Can you work these out from the drawing? Everything is in mm from the part's minimum corner. A direction names the side the tool comes from. Coordinates: 2 decimals unless noted, no trailing zeros. Loops run counter-clockwise (first coordinate to the right, second up) from the corner with the lowest first, then second, coordinate; pieces in that order, holes last. Notation, with made-up numbers: (-31.75, 88) -> (17.25, 88) arc R27 cw to (17.25, 117) -> close; hole circle Ø4 at (-34, 65.5). An arc over 180 degrees is marked (long way). Put each result on its own line as item: value. Start each with the question number.
Item 1: Will these pins go through, and if not, where does the flat tip stop? P1, Ø1.5, axis at x = 14, z = 3, coming from the +Y side; P2, Ø2, axis at x = 8, z = 6, coming from the -Y side.
Item 2: We'd pull the mould along Z, two halves only. Please class the marked faces 1, 2, 3 and 4: pulls with the +Z half, pulls with the -Z half, needs draft (parallel to the pull), parting line crosses it, or undercut.
Item 3: For the marked faces 5 and 6, which set-ups out of +Z, -Z, +X, -X, +Y, -Y let a thin tool reach every point of the face, with its end or its side?
Item 4: If we section it at C-C on y = 11.25: Please give me the cut outline in (x, z) (1 decimal).
Item 5: If we section it at B-B on y = 16.5: Please give me the cut outline in (x, z) (1 decimal).
Item 6: If we section it at D-D on x = 14.75: Please give me the cut outline in (y, z) (1 decimal).
Item 7: Please list where these lines run through material, in increasing order: L1, parallel to Z at x = 2.75, y = 13.5 (1 decimal); L2, parallel to Y at x = 9, z = 0.5 (1 decimal); L3, parallel to X at y = 10.25, z = 4.5 (1 decimal). Write a range as from..to.
Item 8: If we section it at A-A on x = 10.25: Please give me the cut outline in (y, z) (1 decimal).
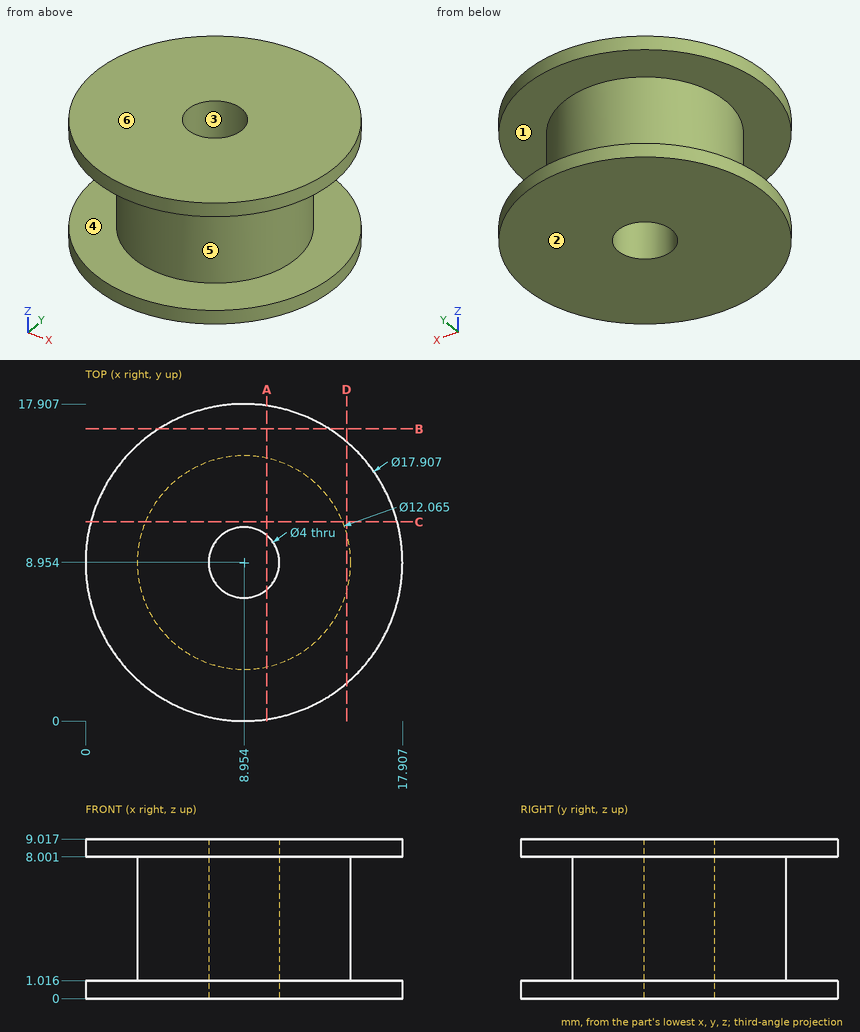
Solutions:
1. P1: y = 13.19
1. P2: y = 2.92
2. face 1: undercut
2. face 2: pulls with the -Z half
2. face 3: needs draft
2. face 4: undercut
3. face 5: none
3. face 6: +Z, +X, -X, +Y, -Y
4. outline: (0.3, 0) -> (17.6, 0) -> (17.6, 1) -> (14.5, 1) -> (14.5, 8) -> (17.6, 8) -> (17.6, 9) -> (0.3, 9) -> (0.3, 8) -> (3.4, 8) -> (3.4, 1) -> (0.3, 1) -> close
5. outline: (4.1, 0) -> (13.8, 0) -> (13.8, 1) -> (4.1, 1) -> close; (4.1, 8) -> (13.8, 8) -> (13.8, 9) -> (4.1, 9) -> close
6. outline: (2.1, 0) -> (15.8, 0) -> (15.8, 1) -> (10.6, 1) -> (10.6, 8) -> (15.8, 8) -> (15.8, 9) -> (2.1, 9) -> (2.1, 8) -> (7.3, 8) -> (7.3, 1) -> (2.1, 1) -> close
7. L1: 0..1, 8..9
7. L2: 0..7, 11..17.9
7. L3: 3.1..7.4, 10.5..14.8
8. outline: (0.1, 0) -> (7.4, 0) -> (7.4, 9) -> (0.1, 9) -> (0.1, 8) -> (3.1, 8) -> (3.1, 1) -> (0.1, 1) -> close; (10.5, 0) -> (17.8, 0) -> (17.8, 1) -> (14.8, 1) -> (14.8, 8) -> (17.8, 8) -> (17.8, 9) -> (10.5, 9) -> close
